Read the model definition and answer for the solid it produces. Units are mm, in the model's axes. Face numbers are marked on the shaded views. Coordinates: 2 decimals unless noted, no trailing zeros. Order: outer loops, then holes, each group sorted by start corner. A loop starts at its lowest first (then second) coordinate and runs counter-clockwise, first axis right, second up. Notation, with made-up numbers: M 45,70.25 L 81,70.25 A26 ccw 81,101.25 Z; hole C 48.5,24.25 d9. An arc over 180 degrees is marked long. Put each result on its own line as item: value.
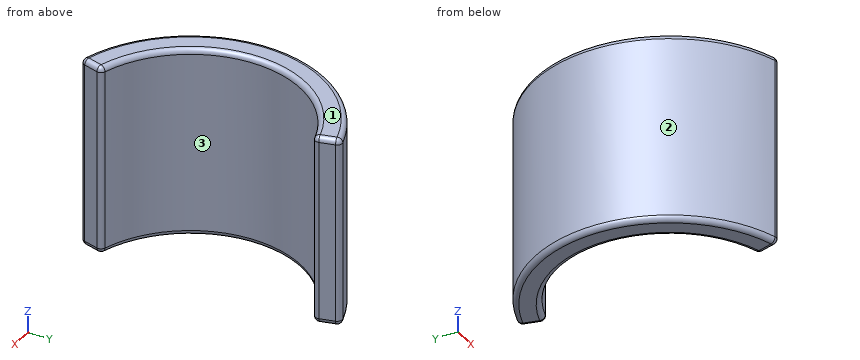
from build123d import *

# Parameters (mm, degrees)
REVOLVE1_START = -9.5
REVOLVE1_DEPTH = 19
FILLET1_R      = 0.5


# Read off the part's stored shape, not the designer's step: Revolve1
with BuildPart() as part:
    # Revolve1 outline → Revolve1 (new body)
    with BuildSketch(Plane.XY.offset(REVOLVE1_START)):
        with BuildLine():
            Line((-2.847009496, 10.625184089), (-3.494057109, 13.039998655))
            ThreePointArc((-3.494057109, 13.039998655), (-13.5, 0), (-3.494057109, -13.039998655))
            Line((-3.494057109, -13.039998655), (-2.847009496, -10.625184089))
            ThreePointArc((-2.847009496, -10.625184089), (-11, 0), (-2.847009496, 10.625184089))
        make_face()
    extrude(amount=REVOLVE1_DEPTH)

    # Fillet1
    fillet1_edges = [part.edges().sort_by_distance(p)[0] for p in [
        (-2.847009496, 10.625184089, 0),
        (-3.170533302, 11.832591372, -9.5),
        (-3.170533302, -11.832591372, -9.5),
        (-3.494057109, -13.039998655, 0),
        (-3.170533302, -11.832591372, 9.5),
        (-2.847009496, -10.625184089, 0),
        (-3.494057109, 13.039998655, 0),
        (-13.5, 0, -9.5),
        (-11, 0, -9.5),
        (-11, 0, 9.5),
        (-13.5, 0, 9.5),
        (-3.170533302, 11.832591372, 9.5),
    ]]
    fillet(fillet1_edges, radius=FILLET1_R)


solid = part.part
Q1. Find section A-A on z = 4.25. Write down the section's boundary in (x, y).
Answers below:
outline: M -3.99,-12.9 A0.5 ccw -3.36,-12.55 L -2.97,-11.1 A0.5 ccw -3.31,-10.49 A11 cw -3.31,10.49 A0.5 ccw -2.97,11.1 L -3.36,12.55 A0.5 ccw -3.99,12.9 A13.5 ccw Z
Q2. For a pull along Y with two mould halves and no side action, classify the marked faces 1, 2 and 3 as +Y half, -Y half, draft (parallel to the pull), parting line (faces both ways), or undercut.
Answers below:
face 1: draft
face 2: parting line
face 3: undercut
Q3. Given pin 1 (5 mm diameter, centred on x = -7, y = 9, fed in from -Z); pin 2 (3 mm diameter, centred on y = 1, z = 1.5, fed in from +X); pin 3 (1.5 mm diameter, centred on y = 7.5, z = -2, fed in from -X); pin 4 (4 mm diameter, centred on y = 3.5, z = -1.5, fed in from +X), each flat-ended and moving along its own axis, determine where each tip first touches the part or whether it passes through.
Answers below:
pin 1: stops at z = -9.5
pin 2: stops at x = -10.71
pin 3: stops at x = -11.69
pin 4: stops at x = -9.53
Q4. Consider line 1 along Y through (x, z) = (-6.75, 7); line 2 along Y through (x, z) = (-10, 8.25); line 3 along X through (y, z) = (6, -6.5). Determine where each line is inside the solid, lowest interval first.
Answers below:
line 1: y = -11.69 to -8.69, 8.69 to 11.69
line 2: y = -9.07 to -4.58, 4.58 to 9.07
line 3: x = -12.09 to -9.22
